from build123d import *
from OCP.BRepFilletAPI import BRepFilletAPI_MakeChamfer

# Parameters (mm, degrees)
SKETCH1_W            = 7.62
SKETCH1_H            = 2.5
BOSS_EXTRUDE1_DEPTH  = 2
CUT_EXTRUDE1_DEPTH   = 9.265252567
SKETCH3_W            = 0.305
SKETCH3_H            = 0.3
CUT_EXTRUDE2_DEPTH   = 2
SKETCH4_W            = 0.305
SKETCH4_H            = 0.3
CUT_EXTRUDE3_DEPTH   = 9.265252567
CUT_EXTRUDE4_DEPTH   = 9.265252567
CUT_EXTRUDE5_DEPTH   = 9.265252567
SKETCH7_W            = 0.305
SKETCH7_H            = 0.3
CUT_EXTRUDE6_DEPTH   = 2
SKETCH8_W            = 0.305
SKETCH8_H            = 0.3
CUT_EXTRUDE7_DEPTH   = 9.265252567
CUT_EXTRUDE8_DEPTH   = 9.265252567
SKETCH10_W           = 0.635
SKETCH10_H           = 0.635
BOSS_EXTRUDE2_DEPTH  = 3.8
SKETCH11_W           = 0.635
SKETCH11_H           = 0.635
BOSS_EXTRUDE3_DEPTH  = 3.8
BOSS_EXTRUDE4_DEPTH  = 0.5
BOSS_EXTRUDE5_DEPTH  = 0.5
BOSS_EXTRUDE6_DEPTH  = 0.5
BOSS_EXTRUDE7_DEPTH  = 0.5
BOSS_EXTRUDE8_DEPTH  = 0.5
BOSS_EXTRUDE9_DEPTH  = 0.5
SKETCH18_W           = 0.635
SKETCH18_H           = 0.635
BOSS_EXTRUDE10_DEPTH = 3.8
SKETCH19_W           = 0.635
SKETCH19_H           = 0.635
BOSS_EXTRUDE11_DEPTH = 6.8
SKETCH20_W           = 0.635
SKETCH20_H           = 0.635
BOSS_EXTRUDE12_DEPTH = 6.8
SKETCH21_W           = 0.635
SKETCH21_H           = 0.635
BOSS_EXTRUDE13_DEPTH = 6.8
DRAFT1_ANGLE         = 45
DRAFT2_ANGLE         = 45
DRAFT3_ANGLE         = 45
DRAFT4_ANGLE         = 45
DRAFT5_ANGLE         = 45
CHAMFER1_SIZE        = 0.007071068
CHAMFER2_SIZE        = 0.207106781
CHAMFER2_SIZE2       = 0.5


with BuildPart() as part:
    # Sketch1 → Boss-Extrude1 (new body)
    with BuildSketch(Plane(origin=(0, 0, 0), x_dir=(-1, 0, 0), z_dir=(0, 0, -1))):
        with Locations((-3.81, 1.25)):
            Rectangle(SKETCH1_W, SKETCH1_H)
    extrude(amount=-BOSS_EXTRUDE1_DEPTH)

    # Sketch2 → Cut-Extrude1 (cut, through all)
    with BuildSketch(Plane.XY.offset(2)):
        Polygon((4.775, 2.5), (5.385, 1.89), (5.385, 2.5), align=None)
    extrude(amount=-CUT_EXTRUDE1_DEPTH, mode=Mode.SUBTRACT)

    # Sketch3 → Cut-Extrude2 (cut)
    with BuildSketch(Plane.XY.offset(2)):
        with Locations((7.4675, 2.35)):
            Rectangle(SKETCH3_W, SKETCH3_H)
    extrude(amount=-CUT_EXTRUDE2_DEPTH, mode=Mode.SUBTRACT)

    # Sketch4 → Cut-Extrude3 (cut, through all)
    with BuildSketch(Plane.XY.offset(2)):
        with Locations((7.4675, 0.15)):
            Rectangle(SKETCH4_W, SKETCH4_H)
    extrude(amount=-CUT_EXTRUDE3_DEPTH, mode=Mode.SUBTRACT)

    # Sketch5 → Cut-Extrude4 (cut, through all)
    with BuildSketch(Plane.XY.offset(2)):
        Polygon((5.385, 0), (5.385, 0.61), (4.775, 0), align=None)
    extrude(amount=-CUT_EXTRUDE4_DEPTH, mode=Mode.SUBTRACT)

    # Sketch6 → Cut-Extrude5 (cut, through all)
    with BuildSketch(Plane.XY.offset(2)):
        Polygon((2.845, 0), (2.235, 0.61), (2.235, 0), align=None)
    extrude(amount=-CUT_EXTRUDE5_DEPTH, mode=Mode.SUBTRACT)

    # Sketch7 → Cut-Extrude6 (cut)
    with BuildSketch(Plane.XY.offset(2)):
        with Locations((0.1525, 0.15)):
            Rectangle(SKETCH7_W, SKETCH7_H)
    extrude(amount=-CUT_EXTRUDE6_DEPTH, mode=Mode.SUBTRACT)

    # Sketch8 → Cut-Extrude7 (cut, through all)
    with BuildSketch(Plane.XY.offset(2)):
        with Locations((0.1525, 2.35)):
            Rectangle(SKETCH8_W, SKETCH8_H)
    extrude(amount=-CUT_EXTRUDE7_DEPTH, mode=Mode.SUBTRACT)

    # Sketch9 → Cut-Extrude8 (cut, through all)
    with BuildSketch(Plane.XY.offset(2)):
        Polygon((2.235, 2.5), (2.235, 1.89), (2.845, 2.5), align=None)
    extrude(amount=-CUT_EXTRUDE8_DEPTH, mode=Mode.SUBTRACT)

    # Sketch10 → Boss-Extrude2 (add)
    with BuildSketch(Plane(origin=(0, 0, 0), x_dir=(-1, 0, 0), z_dir=(0, 0, -1))):
        with Locations((-6.35, 1.25)):
            Rectangle(SKETCH10_W, SKETCH10_H)
    extrude(amount=BOSS_EXTRUDE2_DEPTH)

    # Sketch11 → Boss-Extrude3 (add)
    with BuildSketch(Plane(origin=(0, 0, 0), x_dir=(-1, 0, 0), z_dir=(0, 0, -1))):
        with Locations((-3.81, 1.25)):
            Rectangle(SKETCH11_W, SKETCH11_H)
    extrude(amount=BOSS_EXTRUDE3_DEPTH)

    # Sketch12 → Boss-Extrude4 (add)
    with BuildSketch(Plane(origin=(0, 0, 0), x_dir=(-1, 0, 0), z_dir=(0, 0, -1))):
        with BuildLine():
            Line((-5.6, 0), (-7.1, 0))
            Line((-7.1, 0), (-7.1, 0.75))
            Line((-7.1, 0.75), (-5.6, 0.75))
            add(Edge.make_bspline(
                [(-5.6, 0), (-5.6, 0.25), (-5.6, 0.75)],
                knots=[0, 0, 1, 3, 3], degree=1))
        make_face()
    extrude(amount=BOSS_EXTRUDE4_DEPTH)

    # Sketch13 → Boss-Extrude5 (add)
    with BuildSketch(Plane(origin=(0, 0, 0), x_dir=(-1, 0, 0), z_dir=(0, 0, -1))):
        with BuildLine():
            Line((-3.06, 0), (-4.56, 0))
            Line((-4.56, 0), (-4.56, 0.75))
            Line((-4.56, 0.75), (-3.06, 0.75))
            add(Edge.make_bspline(
                [(-3.06, 0), (-3.06, 0.25), (-3.06, 0.75)],
                knots=[0, 0, 1, 3, 3], degree=1))
        make_face()
    extrude(amount=BOSS_EXTRUDE5_DEPTH)

    # Sketch14 → Boss-Extrude6 (add)
    with BuildSketch(Plane(origin=(0, 0, 0), x_dir=(-1, 0, 0), z_dir=(0, 0, -1))):
        with BuildLine():
            Line((-0.52, 0), (-2.02, 0))
            Line((-2.02, 0), (-2.02, 0.75))
            Line((-2.02, 0.75), (-0.52, 0.75))
            add(Edge.make_bspline(
                [(-0.52, 0), (-0.52, 0.25), (-0.52, 0.75)],
                knots=[0, 0, 1, 3, 3], degree=1))
        make_face()
    extrude(amount=BOSS_EXTRUDE6_DEPTH)

    # Sketch15 → Boss-Extrude7 (add)
    with BuildSketch(Plane(origin=(0, 0, 0), x_dir=(-1, 0, 0), z_dir=(0, 0, -1))):
        with BuildLine():
            Line((-5.6, 1.75), (-7.1, 1.75))
            add(Edge.make_bspline(
                [(-7.1, 2.5), (-7.1, 2.25), (-7.1, 1.75)],
                knots=[-2.2, -2.2, -1.2, 0.8, 0.8], degree=1))
            Line((-7.1, 2.5), (-5.6, 2.5))
            Line((-5.6, 2.5), (-5.6, 1.75))
        make_face()
    extrude(amount=BOSS_EXTRUDE7_DEPTH)

    # Sketch16 → Boss-Extrude8 (add)
    with BuildSketch(Plane(origin=(0, 0, 0), x_dir=(-1, 0, 0), z_dir=(0, 0, -1))):
        with BuildLine():
            Line((-3.06, 1.75), (-4.56, 1.75))
            add(Edge.make_bspline(
                [(-4.56, 2.5), (-4.56, 2.25), (-4.56, 1.75)],
                knots=[-2.2, -2.2, -1.2, 0.8, 0.8], degree=1))
            Line((-4.56, 2.5), (-3.06, 2.5))
            Line((-3.06, 2.5), (-3.06, 1.75))
        make_face()
    extrude(amount=BOSS_EXTRUDE8_DEPTH)

    # Sketch17 → Boss-Extrude9 (add)
    with BuildSketch(Plane(origin=(0, 0, 0), x_dir=(-1, 0, 0), z_dir=(0, 0, -1))):
        with BuildLine():
            Line((-0.52, 1.75), (-2.02, 1.75))
            add(Edge.make_bspline(
                [(-2.02, 2.5), (-2.02, 2.25), (-2.02, 1.75)],
                knots=[-2.2, -2.2, -1.2, 0.8, 0.8], degree=1))
            Line((-2.02, 2.5), (-0.52, 2.5))
            Line((-0.52, 2.5), (-0.52, 1.75))
        make_face()
    extrude(amount=BOSS_EXTRUDE9_DEPTH)

    # Sketch18 → Boss-Extrude10 (add)
    with BuildSketch(Plane(origin=(0, 0, 0), x_dir=(-1, 0, 0), z_dir=(0, 0, -1))):
        with Locations((-1.27, 1.25)):
            Rectangle(SKETCH18_W, SKETCH18_H)
    extrude(amount=BOSS_EXTRUDE10_DEPTH)

    # Sketch19 → Boss-Extrude11 (add)
    with BuildSketch(Plane.XY.offset(2)):
        with Locations((6.35, 1.25)):
            Rectangle(SKETCH19_W, SKETCH19_H)
    extrude(amount=BOSS_EXTRUDE11_DEPTH)

    # Sketch20 → Boss-Extrude12 (add)
    with BuildSketch(Plane.XY.offset(2)):
        with Locations((3.81, 1.25)):
            Rectangle(SKETCH20_W, SKETCH20_H)
    extrude(amount=BOSS_EXTRUDE12_DEPTH)

    # Sketch21 → Boss-Extrude13 (add)
    with BuildSketch(Plane.XY.offset(2)):
        with Locations((1.27, 1.25)):
            Rectangle(SKETCH21_W, SKETCH21_H)
    extrude(amount=BOSS_EXTRUDE13_DEPTH)

    # Draft1
    draft1_faces = [part.faces().sort_by_distance(p)[0] for p in [
        (2.235, 2.195, 1),
        (0.305, 2.35, 1),
    ]]
    draft(draft1_faces, Plane(origin=(0, 2.5, 2), x_dir=(0, 0, 1), z_dir=(0, 1, 0)), DRAFT1_ANGLE)

    # Draft2
    draft2_faces = [part.faces().sort_by_distance(p)[0] for p in [
        (7.315, 2.35, 1),
        (5.385, 2.195, 1),
    ]]
    draft(draft2_faces, Plane(origin=(0, 2.5, 2), x_dir=(0, 0, 1), z_dir=(0, 1, 0)), DRAFT2_ANGLE)

    # Draft3
    draft3_faces = [part.faces().sort_by_distance(p)[0] for p in [
        (5.385, 0.305, 1),
        (7.315, 0.15, 1),
    ]]
    draft(draft3_faces, Plane(origin=(7.62, 0, 2), x_dir=(0, 0, -1), z_dir=(0, -1, 0)), DRAFT3_ANGLE)

    # Draft4
    draft4_faces = [part.faces().sort_by_distance(p)[0] for p in [
        (0.305, 0.15, 1),
        (2.235, 0.305, 1),
    ]]
    draft(draft4_faces, Plane(origin=(7.62, 0, 2), x_dir=(0, 0, -1), z_dir=(0, -1, 0)), DRAFT4_ANGLE)

    # Draft5
    draft5_faces = [part.faces().sort_by_distance(p)[0] for p in [
        (1.27, 0.75, -0.25),
        (3.81, 0.75, -0.25),
        (6.35, 0.75, -0.25),
        (6.35, 1.75, -0.25),
        (3.81, 1.75, -0.25),
        (1.27, 1.75, -0.25),
    ]]
    draft(draft5_faces, Plane(origin=(0, 0, 0), x_dir=(-1, 0, 0), z_dir=(0, 0, -1)), DRAFT5_ANGLE)

    # Chamfer1
    chamfer1_edges = [part.edges().sort_by_distance(p)[0] for p in [
        (2.54, 2.195, 1),
        (5.08, 2.195, 1),
        (5.08, 0.305, 1),
        (2.54, 0.305, 1),
    ]]
    chamfer(chamfer1_edges, length=CHAMFER1_SIZE)

    # Chamfer2: one chamfer whose edges measure the first distance from different faces: ONE call of the kernel's chamfer builder (chamfer() names one face for all edges)
    chamfer2_edges_1 = [part.edges().sort_by_distance(p)[0] for p in [
        (6.6675, 1.25, -3.8),
        (6.35, 0.9325, -3.8),
        (6.0325, 1.25, -3.8),
        (6.35, 1.5675, -3.8),
    ]]
    chamfer2_side_1 = [part.faces().sort_by_distance(p)[0] for p in [
        (6.35, 1.25, -3.8),
    ]]
    chamfer2_edges_2 = [part.edges().sort_by_distance(p)[0] for p in [
        (3.81, 0.9325, -3.8),
        (3.4925, 1.25, -3.8),
        (3.81, 1.5675, -3.8),
        (4.1275, 1.25, -3.8),
    ]]
    chamfer2_side_2 = [part.faces().sort_by_distance(p)[0] for p in [
        (3.81, 1.25, -3.8),
    ]]
    chamfer2_edges_3 = [part.edges().sort_by_distance(p)[0] for p in [
        (1.27, 0.9325, -3.8),
        (0.9525, 1.25, -3.8),
        (1.27, 1.5675, -3.8),
        (1.5875, 1.25, -3.8),
    ]]
    chamfer2_side_3 = [part.faces().sort_by_distance(p)[0] for p in [
        (1.27, 1.25, -3.8),
    ]]
    chamfer2_edges_4 = [part.edges().sort_by_distance(p)[0] for p in [
        (6.0325, 1.25, 8.8),
        (6.35, 0.9325, 8.8),
        (6.6675, 1.25, 8.8),
        (6.35, 1.5675, 8.8),
    ]]
    chamfer2_side_4 = [part.faces().sort_by_distance(p)[0] for p in [
        (6.35, 1.25, 8.8),
    ]]
    chamfer2_edges_5 = [part.edges().sort_by_distance(p)[0] for p in [
        (3.4925, 1.25, 8.8),
        (3.81, 0.9325, 8.8),
        (4.1275, 1.25, 8.8),
        (3.81, 1.5675, 8.8),
    ]]
    chamfer2_side_5 = [part.faces().sort_by_distance(p)[0] for p in [
        (3.81, 1.25, 8.8),
    ]]
    chamfer2_edges_6 = [part.edges().sort_by_distance(p)[0] for p in [
        (0.9525, 1.25, 8.8),
        (1.27, 0.9325, 8.8),
        (1.5875, 1.25, 8.8),
        (1.27, 1.5675, 8.8),
    ]]
    chamfer2_side_6 = [part.faces().sort_by_distance(p)[0] for p in [
        (1.27, 1.25, 8.8),
    ]]
    chamfer2 = BRepFilletAPI_MakeChamfer(part.part.solid().wrapped)
    for e in chamfer2_edges_1:
        chamfer2.Add(CHAMFER2_SIZE, CHAMFER2_SIZE2, e.wrapped, chamfer2_side_1[0].wrapped)  # the first distance lies on this face
    for e in chamfer2_edges_2:
        chamfer2.Add(CHAMFER2_SIZE, CHAMFER2_SIZE2, e.wrapped, chamfer2_side_2[0].wrapped)  # the first distance lies on this face
    for e in chamfer2_edges_3:
        chamfer2.Add(CHAMFER2_SIZE, CHAMFER2_SIZE2, e.wrapped, chamfer2_side_3[0].wrapped)  # the first distance lies on this face
    for e in chamfer2_edges_4:
        chamfer2.Add(CHAMFER2_SIZE, CHAMFER2_SIZE2, e.wrapped, chamfer2_side_4[0].wrapped)  # the first distance lies on this face
    for e in chamfer2_edges_5:
        chamfer2.Add(CHAMFER2_SIZE, CHAMFER2_SIZE2, e.wrapped, chamfer2_side_5[0].wrapped)  # the first distance lies on this face
    for e in chamfer2_edges_6:
        chamfer2.Add(CHAMFER2_SIZE, CHAMFER2_SIZE2, e.wrapped, chamfer2_side_6[0].wrapped)  # the first distance lies on this face
    add(Compound.cast(chamfer2.Shape()), mode=Mode.REPLACE)


solid = part.part
Work out the finished part from the listing and answer in its coordinate system (mm). Give positions to 0.01 mm unless a question says otherwise; leave off trailing zeros. Order: outer loops, then holes, each group sorted by start corner. A loop starts at its lowest first (then second) coordinate and runs counter-clockwise, first axis right, second up. Notation, with made-up numbers: (-31.75, 86) -> (-18.75, 86) arc R20 ccw to (-18.75, 92) -> close; hole circle Ø9 at (-31, -13.5). An arc over 180 degrees is marked (long way). One line per item, written item: value.
Item 1: Straight lines are drawn through the part: probe 1 along X at (y, z) = (1.05, 4); probe 2 along Z at (x, y) = (3, 1.1); probe 3 along Z at (x, y) = (3.25, 2.3). For each, find the intervals that lie inside material, in ascending order.
Answer sheet:
probe 1: 0.95 to 1.59, 3.49 to 4.13, 6.03 to 6.67
probe 2: 0 to 2
probe 3: -0.5 to 2
Item 2: Find section A-A, the plane z = 7. Give the vertices of the cut face in (x, y), plus the area to 3 significant figures.
Answer sheet:
outline: (0.95, 0.93) -> (1.59, 0.93) -> (1.59, 1.57) -> (0.95, 1.57) -> close; (3.49, 0.93) -> (4.13, 0.93) -> (4.13, 1.57) -> (3.49, 1.57) -> close; (6.03, 0.93) -> (6.67, 0.93) -> (6.67, 1.57) -> (6.03, 1.57) -> close
area: 1.21 mm²
Item 3: Determine the mould class of faces 1 (the flat face through (3, 1, 0)), 2 (the flat face through (7.62, 1, 1)), 3 (the flat face through (6, 2.5, 1)) for opening direction X: released by +X, released by -X, zero draft, split by the parting line, or undercut.
Answer sheet:
face 1: undercut
face 2: released by +X
face 3: zero draft
Item 4: Flat-ended cylindrical pins translate along their axes: P1, Ø0.7, axis at x = 1.5, z = 5, coming from the +Y side; P2, Ø1.5, axis at y = 1, z = 3.5, coming from the -X side; P3, Ø0.5, axis at y = 1, z = 4, coming from the +X side. Find the tip coordinate at first contact, or state that the pin passes through.
Answer sheet:
P1: y = 1.57
P2: x = 0.95
P3: x = 6.67
